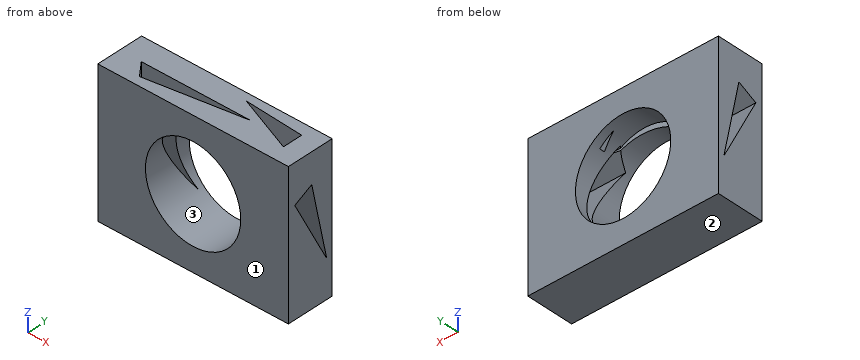
```python
from build123d import *

# Parameters (mm, degrees)
F0_W     = 101.6
F0_H     = 76.2
F1_DEPTH = 25.4
F2_R     = 25.4
F3_DEPTH = 25.401
F5_DEPTH = 19.05
F7_DEPTH = 19.05
F9_DEPTH = 101.601


with BuildPart() as f1:
    # F0 (on Front) → F1 (new body)
    with BuildSketch(Plane.XZ):
        with Locations((50.8, 38.1)):
            Rectangle(F0_W, F0_H)
    extrude(amount=F1_DEPTH)

    # F2 (on face) → F3 (cut, through all)
    with BuildSketch(Plane.XZ.offset(25.4)):
        with Locations((50.8, 38.1)):
            Circle(F2_R)
    extrude(amount=-F3_DEPTH, mode=Mode.SUBTRACT)

    # F4 (on face) → F5 (cut)
    with BuildSketch(Plane.XY.offset(76.2)):
        Polygon((69.784895, -12.7), (11.520899, -12.7), (17.740097, -20.550709), align=None)
    extrude(amount=-F5_DEPTH, mode=Mode.SUBTRACT)

    # F6 (on face) → F7 (cut)
    with BuildSketch(Plane.XY.offset(76.2)):
        Polygon((59.600811, -4.206988), (91.207154, -16.983436), (91.207154, -6.414911), align=None)
    extrude(amount=-F7_DEPTH, mode=Mode.SUBTRACT)

    # F8 (on face) → F9 (cut, through all)
    with BuildSketch(Plane.YZ.offset(101.6)):
        Polygon((-3.176994, 19.873125), (-11.888587, 60.30136), (-21.700324, 55.405151), align=None)
    extrude(amount=-F9_DEPTH, mode=Mode.SUBTRACT)


solid = f1.part
```
Geometry: final body of the model. Coordinates: model frame, mm. Face numbers are marked on the shaded views. Coordinates: 2 decimals unless noted, no trailing zeros. Order: outer loops, then holes, each group sorted by start corner. A loop starts at its lowest first (then second) coordinate and runs counter-clockwise, first axis right, second up. Notation, with made-up numbers: (-3, -5) - (16, -5) arc R24 cw to (16, 9) - close; hole circle Ø1 at (82.25, 22.25). An arc over 180 degrees is marked (long way). Write each question's results on one line, items separated by ' | '.
(1) Section query A-A, the plane x = 93.5. Return the cut outline in (y, z), plus the area to 3 significant figures.
Values found:
outline: (-25.4, 0) - (0, 0) - (0, 76.2) - (-25.4, 76.2) - close; hole (-21.7, 55.41) - (-3.18, 19.87) - (-11.89, 60.3) - close | area: 1,720 mm²
(2) Section query B-B, the plane x = 72.5. Return the cut outline in (y, z).
Values found:
outline: (-25.4, 0) - (0, 0) - (0, 24.9) - (-4.26, 24.9) - (-3.18, 19.87) - (-5.8, 24.9) - (-25.4, 24.9) - close; (-25.4, 51.3) - (-19.56, 51.3) - (-21.7, 55.41) - (-11.89, 60.3) - (-9.95, 51.3) - (0, 51.3) - (0, 76.2) - (-5.11, 76.2) - (-5.11, 57.15) - (-9.42, 57.15) - (-9.42, 76.2) - (-25.4, 76.2) - close
(3) Section query D-D, the plane z = 51.5. Return the cut outline in (x, y), plus the area to 3 significant figures.
Values found:
outline: (0, -25.4) - (29.22, -25.4) - (29.22, -19.66) - (0, -19.66) - close; (0, -9.99) - (29.22, -9.99) - (29.22, 0) - (0, 0) - close; (72.38, -25.4) - (101.6, -25.4) - (101.6, -19.66) - (72.38, -19.66) - close; (72.38, -9.99) - (101.6, -9.99) - (101.6, 0) - (72.38, 0) - close | area: 919 mm²
(4) Mould query, pull axis Z, two halves, no side actions, for the marked faces 1, 2 and 3. Classes: +Z half, -Z half, draft (parallel to the pull), parting line (faces both ways), or undercut.
Values found:
face 1: draft | face 2: -Z half | face 3: undercut
(5) Line query: line 1 (Z direction, x = 50.8, y = -18); line 2 (X direction, y = -6.75, z = 38.1); line 3 (Y direction, x = 77.5, z = 55.5). Output: solid intervals per line, ascending. Write a range as [from, to].
Values found:
line 1: z = [0, 12.7], [63.5, 76.2] | line 2: x = [0, 25.4], [76.2, 101.6] | line 3: y = [-25.4, -21.51], [-10.85, 0]
(6) Section query C-C, the plane y = -9.5. Return the cut outline in (x, z), plus the area to 3 significant figures.
Values found:
outline: (0, 0) - (101.6, 0) - (101.6, 32) - (75.46, 32) arc R25.4 cw to (26.14, 32) - (0, 32) - close; (0, 49.22) - (27.96, 49.22) arc R25.4 cw to (73.64, 49.22) - (101.6, 49.22) - (101.6, 76.2) - (91.21, 76.2) - (91.21, 57.15) - (72.69, 57.15) - (72.69, 76.2) - (0, 76.2) - close | area: 4,470 mm²
